```python
from build123d import *

# Parameters (mm, degrees)
F0_R     = 23.25
F0_R_2   = 13
F1_DEPTH = 8


with BuildPart() as f1:
    # F0 (on Front) → F1 (new body)
    with BuildSketch(Plane.XZ):
        with BuildLine():
            Line((40, -52.5), (40, 62.5))
            Line((40, 62.5), (-40, 62.5))
            Line((-40, 62.5), (-40, -52.5))
            ThreePointArc((-40, -52.5), (-37.071068, -59.571068), (-30, -62.5))
            Line((-30, -62.5), (30, -62.5))
            ThreePointArc((30, -62.5), (37.071068, -59.571068), (40, -52.5))
        make_face()
        with Locations((0, -27.5)):
            Circle(F0_R, mode=Mode.SUBTRACT)
        with Locations((0, 37.5)):
            Circle(F0_R_2, mode=Mode.SUBTRACT)
    extrude(amount=F1_DEPTH)


solid = f1.part
```
Can you work these out from the model? Positions are in its coordinate system, mm. Coordinates: 2 decimals unless noted, no trailing zeros. Order: outer loops, then holes, each group sorted by start corner. A loop starts at its lowest first (then second) coordinate and runs counter-clockwise, first axis right, second up. Notation, with made-up numbers: (3, -20.75) -> (12, -20.75) arc R14 ccw to (12, -16.75) -> close; hole circle Ø8 at (75.25, 42). An arc over 180 degrees is marked (long way). Write each question's results on one line, items separated by ' | '.
Item 1: I want a section at B-B, the plane z = -27.5. Write out the boundary of the cut face in (x, y).
Results are:
outline: (-40, -8) -> (-23.25, -8) -> (-23.25, 0) -> (-40, 0) -> close; (23.25, -8) -> (40, -8) -> (40, 0) -> (23.25, 0) -> close
Item 2: If we mould it in two halves opening along X, with no side actions, what happens to faces 1 (the face through (-18.45, -3.94, -41.65)), 2 (the face through (-37.15, -3.94, -59.49)), 3 (the face through (1, -4, 62.5))? For each: +X half, -X half, draft (parallel to the pull), parting line (faces both ways), or undercut.
Results are:
face 1: undercut | face 2: -X half | face 3: draft
Item 3: If I drill on line 1 along Z through (x, y) = (0, -2); line 2 along Z through (x, y) = (-3, -4); line 3 along X through (y, z) = (-4, 40.5), over which ranges is the centre line in solid material (lowest first)?
Results are:
line 1: -62.5 to -50.75, -4.25 to 24.5, 50.5 to 62.5 | line 2: -62.5 to -50.56, -4.44 to 24.85, 50.15 to 62.5 | line 3: -40 to -12.65, 12.65 to 40
Item 4: I want a section at C-C, the plane y = -2.25. Write out the boundary of the cut face in (x, z).
Results are:
outline: (-40, -52.5) arc R10 ccw to (-30, -62.5) -> (30, -62.5) arc R10 ccw to (40, -52.5) -> (40, 62.5) -> (-40, 62.5) -> close; hole circle Ø46.5 at (0, -27.5); hole circle Ø26 at (0, 37.5)
Item 5: I want a section at D-D, the plane z = 37.5. Write out the boundary of the cut face in (x, y), then the cut area to 3 significant figures.
Results are:
outline: (-40, -8) -> (-13, -8) -> (-13, 0) -> (-40, 0) -> close; (13, -8) -> (40, -8) -> (40, 0) -> (13, 0) -> close | area: 432 mm²
Item 6: I want a section at A-A, the plane x = 0. Write out the boundary of the cut face in (y, z), then the cut area to 3 significant figures.
Results are:
outline: (-8, -62.5) -> (0, -62.5) -> (0, -50.75) -> (-8, -50.75) -> close; (-8, -4.25) -> (0, -4.25) -> (0, 24.5) -> (-8, 24.5) -> close; (-8, 50.5) -> (0, 50.5) -> (0, 62.5) -> (-8, 62.5) -> close | area: 420 mm²
